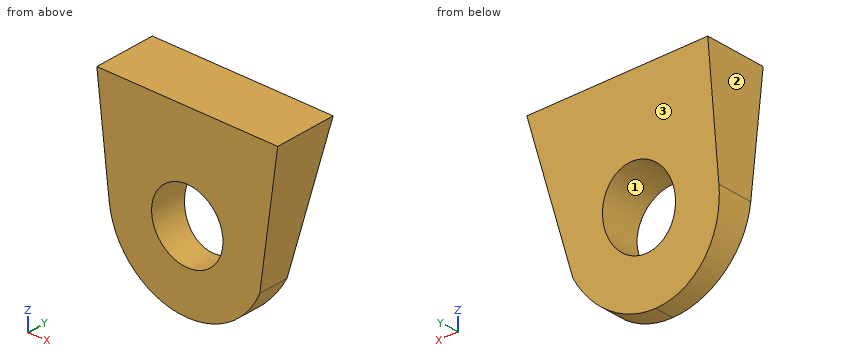
```python
from build123d import *

# Parameters (mm, degrees)
SKETCH1_R               = 1.905
BOSS_EXTRUDE3_DEPTH     = 3.302
BOUNDARY_CUT1_START     = 3.213111109
BOUNDARY_CUT1_OUTLINE_W = 12
BOUNDARY_CUT1_OUTLINE_H = 13
BOUNDARY_CUT1_DEPTH     = 2.224461537


# Read off the part's stored shape, not the designer's step: Boundary-Cut1
with BuildPart() as part:
    # Sketch1 → Boss-Extrude3 (new body)
    with BuildSketch(Plane(origin=(0, 0, 0), x_dir=(1, 0, 0), z_dir=(0, 1, 0))):
        with BuildLine():
            Line((0, 0), (-4.826, 0))
            Line((-4.826, 0), (-4.165178795, 5.925506842))
            ThreePointArc((-4.165178795, 5.925506842), (-2.7944349, 8.584397923), (0, 9.652))
            ThreePointArc((0, 9.652), (2.321880516, 8.950033085), (3.865959408, 7.079282688))
            Line((3.865959408, 7.079282688), (4.826, 0))
            Line((4.826, 0), (0, 0))
        make_face()
        with Locations(Location((0, 5.461, 0), (0, 0, 90))):
            Circle(SKETCH1_R, mode=Mode.SUBTRACT)
    extrude(amount=BOSS_EXTRUDE3_DEPTH)

    # Boundary-Cut1 outline → Boundary-Cut1 (cut)
    with BuildSketch(Plane(origin=(0, 0, 0), x_dir=(1, 0, 0), z_dir=(0, 0.9730802874900094, -0.23046638387921312)).offset(BOUNDARY_CUT1_START)):
        with Locations((0, 4.5)):
            Rectangle(BOUNDARY_CUT1_OUTLINE_W, BOUNDARY_CUT1_OUTLINE_H)
    extrude(amount=BOUNDARY_CUT1_DEPTH, mode=Mode.SUBTRACT)


solid = part.part
```
Could you check a few things on this model? Use its own coordinates, in mm. Face numbers are marked on the shaded views. Round coordinates to 2 decimals unless told otherwise and drop trailing zeros. Loops run counter-clockwise (first coordinate to the right, second up) from the corner with the lowest first, then second, coordinate; pieces in that order, holes last. Notation, with made-up numbers: (58, 36.5) -> (111, 36.5) arc R17 cw to (111, 62.5) -> close; hole circle Ø4 at (79.25, -26.75). An arc over 180 degrees is marked (long way). Put each result on its own line as item: value.
Q1. I want a section at B-B on x = 1. Write out the boundary of the cut face in (y, z).
Checks:
outline: (0, -9.53) -> (1.04, -9.53) -> (1.62, -7.08) -> (0, -7.08) -> close; (0, -3.84) -> (2.39, -3.84) -> (3.3, 0) -> (0, 0) -> close
Q2. Please list where these lines run through material, in increasing order: line 1 (X direction, y = 0.3, z = -4.5); line 2 (X direction, y = 1.8, z = -3.75); line 3 (Z direction, x = 0, y = 1.7). Write a range as from..to.
Checks:
line 1: -4.32..-1.64, 1.64..4.22
line 2: -4.41..-0.84, 0.84..4.32
line 3: -3.56..0
Q3. Thinking about a two-plate mould opening in X: for the marked faces 1, 2 and 3, which applies, pulls with the +X half, pulls with the -X half, needs draft (parallel to the pull), parting line crosses it, or undercut?
Checks:
face 1: undercut
face 2: pulls with the -X half
face 3: needs draft
Q4. I want a section at C-C on y = 0.4. Write out the boundary of the cut face in (x, z) (1 decimal), and give its area (3 significant figures).
Checks:
outline: (-4.8, 0) -> (-4.2, -5.9) arc R4.2 ccw to (3.9, -7.1) -> (4.8, 0) -> close; hole circle Ø3.8 at (0, -5.5)
area: 65.0 mm2
Q5. I want a section at D-D on x = 4.25. Write out the boundary of the cut face in (y, z).
Checks:
outline: (0, -4.25) -> (2.3, -4.25) -> (3.3, 0) -> (0, 0) -> close
Q6. For pin 1 Ø5 at (x, z) = (0, -5.461) entering from +Y, with a flat end and sliding along its axis, tell me the tip position at first contact or that it passes through.
Checks:
pin 1: y = 2.6
Q7. I want a section at A-A on z = -6.75. Write out the boundary of the cut face in (x, y).
Checks:
outline: (-3.99, 0) -> (-1.4, 0) -> (-1.4, 1.7) -> (-3.99, 1.7) -> close; (1.4, 0) -> (3.91, 0) -> (3.91, 1.7) -> (1.4, 1.7) -> close
